```python
from build123d import *

# Parameters (mm, degrees)
F0_R     = 3.5
F0_R_2   = 1.6
F1_DEPTH = 1.5
F2_R     = 0.5
F3_SIZE  = 0.3


with BuildPart() as f1:
    # F0 (on Top) → F1 (new body)
    with BuildSketch(Plane.XY):
        Circle(F0_R)
        Circle(F0_R_2, mode=Mode.SUBTRACT)
    extrude(amount=F1_DEPTH)

    # F2
    f2_edges = [f1.edges().sort_by_distance(p)[0] for p in [
        (1.6, 0, 0.75),
        (-1.6, 0, 0),
        (-1.6, 0, 1.5),
    ]]
    fillet(f2_edges, radius=F2_R)

    # F3
    f3_edges = [f1.edges().sort_by_distance(p)[0] for p in [
        (3.5, 0, 0.75),
        (-3.5, 0, 0),
        (-3.5, 0, 1.5),
    ]]
    chamfer(f3_edges, length=F3_SIZE)


solid = f1.part
```
For this review, take the finished solid that the model builds, in its own axes (mm). Coordinates: 2 decimals unless noted, no trailing zeros. Loops run counter-clockwise (first coordinate to the right, second up) from the corner with the lowest first, then second, coordinate; pieces in that order, holes last. Notation, with made-up numbers: (54.25, 32.25) - (66.25, 32.25) arc R28 ccw to (66.25, 59.25) - close; hole circle Ø10 at (28.5, -39). An arc over 180 degrees is marked (long way). Use one line per item in the form item = value. Start each with the question number.
1) Take a section at C-C (z = 0.7). State the section outline as (x, y) points, plus the area to 3 significant figures.
2) Draft analysis for pull direction X (two halves, no side actions). For faces 1 (the face through (3.233, -1.341, 0.744)), 2 (the face through (-1.27, -0.97, 0.75)), state which applies: released by +X, released by -X, zero draft, split by the parting line, or undercut.
3) To check wall thickness, follow probe 1 along Y at (x, z) = (0, 0.85); probe 2 along Y at (x, z) = (1.25, 1.3); probe 3 along X at (y, z) = (1.75, 1). State the ranges of each line that lie inside material, in increasing order. Write a range as from..to.
4) Take a section at A-A (y = 0). State the section outline as (x, z) points, plus the area to 3 significant figures.
From the geometry:
q1.outline = circle Ø7 at (0, 0); hole circle Ø3.2 at (0, 0)
q1.area = 30.4 mm2
q2.face_1 = split by the parting line
q2.face_2 = undercut
q3.probe_1 = -3.5..-1.6, 1.6..3.5
q3.probe_2 = -3.16..-1.15, 1.15..3.16
q3.probe_3 = -3.03..3.03
q4.outline = (-3.5, 0.3) - (-3.2, 0) - (-2.1, 0) arc R0.5 ccw to (-1.6, 0.5) - (-1.6, 1) arc R0.5 ccw to (-2.1, 1.5) - (-3.2, 1.5) - (-3.5, 1.2) - close; (1.6, 0.5) arc R0.5 ccw to (2.1, 0) - (3.2, 0) - (3.5, 0.3) - (3.5, 1.2) - (3.2, 1.5) - (2.1, 1.5) arc R0.5 ccw to (1.6, 1) - close
q4.area = 5.31 mm2
